Read the model definition and answer for the solid it produces. Units are mm, in the model's axes. A direction names the side the tool comes from. Coordinates: 2 decimals unless noted, no trailing zeros. Write each loop counter-clockwise with the first axis right and the second up, starting at its lowest first coordinate (ties: lowest second). Pieces come first, ordered by that corner, then holes. Notation, with made-up numbers: (86.5, -33.75) -> (139.5, -33.75) arc R19 cw to (139.5, -3.75) -> close; hole circle Ø3 at (-11, -13). An arc over 180 degrees is marked (long way). Write item = value, one per line. Start each with the question number.
1) Section D-D (y = 12.5) is taken. Determine the outline of the cut face in (x, z), plus the area to 3 significant figures.
2) A tool of negligible diameter and unlimited length cuts with its end or side. For faces 3 (the face through (49, 0, 4)), 4 (the face through (50, 10, 2)), 5 (the face through (5, -13, 2)), from which of +Z, -Z, +X, -X, +Y, -Y can it reach the whole face along a straight path? Write none if from no direction.
3) For a pull along X with two mould halves and no side action, classify faces 1 (the face through (49, 0, 0)), 2 (the face through (12, -16, 2)) as released by +X, released by -X, zero draft, split by the parting line, or undercut.
4) Section C-C (y = -1.5) is taken. Determine the outline of the cut face in (x, z).
5) Section A-A (x = 100) is taken. Determine the outline of the cut face in (y, z).
6) Find the intervals of material crossed by line 1 along X through (y, z) = (5, 2.4) (3 decimals); line 2 along Y through (x, z) = (100, 1.65); line 3 along X through (y, z) = (2, 1.65), in increasing order. Write a range as from..to.
7) Flat-ended cylindrical pins translate along their axes: pin 1 Ø1.2 at (y, z) = (-12, 1) entering from +X; pin 2 Ø1.5 at (x, z) = (89, 2.5) entering from -Y. Find the tip coordinate at first contact, or state that the pin passes through.
from build123d import *

# Parameters (mm, degrees)
SKETCH1_R           = 20
BOSS_EXTRUDE1_DEPTH = 4
BOSS_EXTRUDE2_DEPTH = 4
SKETCH4_R           = 8
CUT_EXTRUDE1_DEPTH  = 4
SKETCH5_W           = 10
SKETCH5_H           = 19.132811744
CUT_EXTRUDE3_DEPTH  = 4
SKETCH6_R           = 6.05
CUT_EXTRUDE4_DEPTH  = 4


with BuildPart() as part:
    # Sketch1 → Boss-Extrude1 (new body)
    with BuildSketch(Plane.XY):
        Circle(SKETCH1_R)
    extrude(amount=BOSS_EXTRUDE1_DEPTH)

    # Sketch3 → Boss-Extrude2 (add)
    with BuildSketch(Plane.XY):
        with BuildLine():
            ThreePointArc((120, 0), (105.176380902, 19.318516526), (82.679491924, 10))
            Line((82.679491924, 10), (100, 10))
            Line((100, 10), (100, 0))
            Line((100, 0), (100, -10))
            Line((100, -10), (82.679491924, -10))
            ThreePointArc((82.679491924, -10), (105.176380902, -19.318516526), (120, 0))
        make_face()
        with BuildLine():
            Line((100, 10), (82.679491924, 10))
            ThreePointArc((82.679491924, 10), (80, 0), (82.679491924, -10))
            Line((82.679491924, -10), (100, -10))
            Line((100, -10), (100, 0))
            Line((100, 0), (100, 10))
        make_face()
        with BuildLine():
            Line((82.679491924, 10), (0, 10))
            Line((0, 10), (0, 0))
            Line((0, 0), (0, -10))
            Line((0, -10), (82.679491924, -10))
            ThreePointArc((82.679491924, -10), (80, 0), (82.679491924, 10))
        make_face()
    extrude(amount=BOSS_EXTRUDE2_DEPTH)

    # Sketch4 → Cut-Extrude1 (cut)
    with BuildSketch(Plane.XY):
        Circle(SKETCH4_R)
    extrude(amount=CUT_EXTRUDE1_DEPTH, mode=Mode.SUBTRACT)

    # Sketch5 → Cut-Extrude3 (cut)
    with BuildSketch(Plane.XY):
        with Locations((0, -14.406019059)):
            Rectangle(SKETCH5_W, SKETCH5_H)
    extrude(amount=CUT_EXTRUDE3_DEPTH, mode=Mode.SUBTRACT)

    # Sketch6 → Cut-Extrude4 (cut)
    with BuildSketch(Plane.XY):
        with Locations((100, 0)):
            Circle(SKETCH6_R)
    extrude(amount=CUT_EXTRUDE4_DEPTH, mode=Mode.SUBTRACT)


solid = part.part
Answer key:
q1.outline = (-15.61, 0) -> (15.61, 0) -> (15.61, 4) -> (-15.61, 4) -> close; (84.39, 0) -> (115.61, 0) -> (115.61, 4) -> (84.39, 4) -> close
q1.area = 250 mm^2
q2.face_3 = +Z, +X, -X, +Y, -Y
q2.face_4 = +Z, -Z, +Y
q2.face_5 = +Z, -Z, -Y
q3.face_1 = zero draft
q3.face_2 = undercut
q4.outline = (-19.94, 0) -> (-7.86, 0) -> (-7.86, 4) -> (-19.94, 4) -> close; (7.86, 0) -> (94.14, 0) -> (94.14, 4) -> (7.86, 4) -> close; (105.86, 0) -> (119.94, 0) -> (119.94, 4) -> (105.86, 4) -> close
q5.outline = (-20, 0) -> (-6.05, 0) -> (-6.05, 4) -> (-20, 4) -> close; (6.05, 0) -> (20, 0) -> (20, 4) -> (6.05, 4) -> close
q6.line_1 = -19.365..-6.245, 6.245..96.594, 103.406..119.365
q6.line_2 = -20..-6.05, 6.05..20
q6.line_3 = -19.9..-7.75, 7.75..94.29, 105.71..119.9
q7.pin_1 = 116.43
q7.pin_2 = -17.17
